from build123d import *

# Parameters (mm, degrees)
SKETCH1_W                = 160
SKETCH1_H                = 100
BOSS_EXTRUDE2_DEPTH      = 24
SKETCH3_W                = 52
SKETCH3_H                = 10
CUT_EXTRUDE1_DEPTH       = 160
SKETCH4_W                = 12
SKETCH4_H                = 12
CUT_EXTRUDE2_DEPTH       = 160
SKETCH5_W                = 12
SKETCH5_H                = 12
CUT_EXTRUDE3_DEPTH       = 160
SKETCH6_R                = 15
BOSS_EXTRUDE3_DEPTH      = 76
BOSS_EXTRUDE4_DEPTH      = 6
BOSS_EXTRUDE4_DEPTH_BACK = 6


with BuildPart() as part:
    # Sketch1 → Boss-Extrude2 (new body)
    with BuildSketch(Plane(origin=(0, 0, 0), x_dir=(1, 0, 0), z_dir=(0, 1, 0))):
        Rectangle(SKETCH1_W, SKETCH1_H)
    extrude(amount=BOSS_EXTRUDE2_DEPTH)

    # Sketch3 → Cut-Extrude1 (cut)
    with BuildSketch(Plane(origin=(80, 0, 0), x_dir=(0, 0, -1), z_dir=(1, 0, 0))):
        with Locations((0, 5)):
            Rectangle(SKETCH3_W, SKETCH3_H)
    extrude(amount=-CUT_EXTRUDE1_DEPTH, mode=Mode.SUBTRACT)

    # Sketch4 → Cut-Extrude2 (cut)
    with BuildSketch(Plane(origin=(80, 0, 0), x_dir=(0, 0, -1), z_dir=(1, 0, 0))):
        with Locations((44, 18)):
            Rectangle(SKETCH4_W, SKETCH4_H)
    extrude(amount=-CUT_EXTRUDE2_DEPTH, mode=Mode.SUBTRACT)

    # Sketch5 → Cut-Extrude3 (cut)
    with BuildSketch(Plane(origin=(80, 0, 0), x_dir=(0, 0, -1), z_dir=(1, 0, 0))):
        with Locations((-44, 18)):
            Rectangle(SKETCH5_W, SKETCH5_H)
    extrude(amount=-CUT_EXTRUDE3_DEPTH, mode=Mode.SUBTRACT)

    # Sketch6 → Boss-Extrude3 (add)
    with BuildSketch(Plane(origin=(0, 0, -38), x_dir=(-1, 0, 0), z_dir=(0, 0, -1))):
        with BuildLine():
            Line((80, 24), (80, 66))
            ThreePointArc((80, 66), (50, 96), (20, 66))
            Line((20, 66), (20, 24))
            Line((20, 24), (80, 24))
        make_face()
        with Locations((50, 66)):
            Circle(SKETCH6_R, mode=Mode.SUBTRACT)
    extrude(amount=-BOSS_EXTRUDE3_DEPTH)

    # Sketch7 → Boss-Extrude4 (add, two sides: drawn at the far end of the back side and taken through both)
    with BuildSketch(Plane.XY.offset(-BOSS_EXTRUDE4_DEPTH_BACK)):
        with BuildLine():
            Line((-20, 24), (80, 24))
            Line((80, 24), (-29.728388886, 88.114741301))
            ThreePointArc((-29.728388886, 88.114741301), (-22.539589101, 78.079976543), (-20, 66))
            Line((-20, 66), (-20, 24))
        make_face()
    extrude(amount=BOSS_EXTRUDE4_DEPTH + BOSS_EXTRUDE4_DEPTH_BACK)


solid = part.part
Verification items for the finished model (mm, model axes). A direction names the side the tool comes from. Give positions to 0.01 mm unless a question says otherwise; leave off trailing zeros. Write each loop counter-clockwise with the first axis right and the second up, starting at its lowest first coordinate (ties: lowest second). Pieces come first, ordered by that corner, then holes. Notation, with made-up numbers: M 40,54 L 81,54 A21 ccw 81,85 Z; hole C -3.5,18.5 d10. An arc over 180 degrees is marked long. Put each result on its own line as item: value. Start each with the question number.
1. Draft check along X on faces 4 (the face through (-46.748, 51.357, -0.532)), 5 (the face through (1, 5, -26)), 6 (the face through (-20, 45, 22)), 7 (the face through (-50.66, 95.993, -0.532)). Enter one of: +X half, -X half, draft (parallel to the pull), parting line (faces both ways), or undercut.
2. Section check A-A (x = -50). Record the cut outline in (y, z).
3. Set-up check for faces 1 (the face through (9, 42, -6)), 2 (the face through (1, 12, 44)), 3 (the face through (9, 42, 6)): record each of +Z, -Z, +X, -X, +Y, -Y from which the full face is reachable in a straight line by a thin tool's end or side.
4. Section check D-D (z = 8). Record the cut outline in (x, y).
5. Section check B-B (z = -36). Record the cut outline in (x, y), and give its area (3 significant figures).
6. Scan lines: line 1 along Y through (x, z) = (-50, -13.5); line 2 along Z through (x, y) = (18, 45.5); line 3 along Y through (x, z) = (11.5, -22). Record each from-to range of solid material in increasing order. Write a range as [from, to].
7. Go/stop test with flat-tipped pins: pin 1 Ø3 at (y, z) = (73.5, 38) entering from -X; pin 2 Ø12 at (x, z) = (-45, 14.5) entering from +Y; pin 3 Ø19 at (x, y) = (39.5, 52) entering from +Z. Record where each tip stops, or that it passes through.
8. Section check C-C (y = 74). Record the cut outline in (x, z).
Answer list:
1. face 4: undercut
1. face 5: draft
1. face 6: +X half
1. face 7: parting line
2. outline: M 0,-50 L 12,-50 L 12,-38 L 51,-38 L 51,38 L 12,38 L 12,50 L 0,50 L 0,26 L 10,26 L 10,-26 L 0,-26 Z; M 81,-38 L 96,-38 L 96,38 L 81,38 Z
3. face 1: -Z, +X, +Y
3. face 2: +Z, +X, -X, +Y
3. face 3: +Z, +X, +Y
4. outline: M -80,10 L 80,10 L 80,24 L -20,24 L -20,66 A30 ccw -80,66 Z; hole C -50,66 d30
5. outline: M -80,0 L 80,0 L 80,24 L -20,24 L -20,66 A30 ccw -80,66 Z; hole C -50,66 d30
5. area: 7,070 mm2
6. line 1: [10, 51], [81, 96]
6. line 2: [-6, 6]
6. line 3: [10, 24]
7. pin 1: x = -79.39
7. pin 2: y = 96
7. pin 3: z = 6
8. outline: M -78.91,-38 L -62.69,-38 L -62.69,38 L -78.91,38 Z; M -37.31,-38 L -21.09,-38 L -21.09,-6 L -5.57,-6 L -5.57,6 L -21.09,6 L -21.09,38 L -37.31,38 Z
